For this review, take the finished solid that the model builds, in its own axes (mm). Face numbers are marked on the shaded views. Coordinates: 2 decimals unless noted, no trailing zeros. Loops run counter-clockwise (first coordinate to the right, second up) from the corner with the lowest first, then second, coordinate; pieces in that order, holes last. Notation, with made-up numbers: M 32,42 L 74,42 A34 cw 74,77 Z; hole C 42.25,16.25 d6. An arc over 180 degrees is marked long. Put each result on its own line as item: value.
Autodesk Inventor part; units mm, degrees
ref_plane "B1_XY" through (5.5, 0, 13.5) normal (1, 0, 0) x (0, 0, -1)
ref_plane "B1_YZ" through (5.5, 0, 13.5) normal (0, 0, -1) x (0, 1, 0)
ref_plane "B1_ZX" through (5.5, 0, 13.5) normal (0, 1, 0) x (1, 0, 0)
sketch "Sketch_1" plane through (0, 0, 0) normal (0, 0, 1) x (1, 0, 0)
  line L0 (5.5, 0) -> (-5.5, 0)
  line L1 (-5.5, 13.5) -> (-5.5, 9)
  line L2 (-5.5, 9) -> (-4.688, 8.188)
  line L3 (-4.688, 8.188) -> (4.688, 8.188)
  line L4 (4.688, 8.188) -> (5.5, 9)
  line L5 (5.5, 9) -> (5.5, 13.5)
  line L6 (5.5, 13.5) -> (3.7102, 16.6)
  line L7 (3.7102, 16.6) -> (-3.7102, 16.6)
  line L8 (-3.7102, 16.6) -> (-5.5, 13.5)
revolve "Revolution1" add sketch "Sketch_1" angle 360 about axis through (5.5, 0, 0) along (1, 0, 0)
thread "Thread1"
sketch "Sketch_2" plane through (0, 0, 0) normal (1, 0, 0) x (0, 1, 0)
  circle A0 centre (0, 0) radius 50
  line L0 (-7.7942, 13.5) -> (-15.5885, 0)
  line L1 (-15.5885, 0) -> (-7.7942, -13.5)
  line L2 (-7.7942, -13.5) -> (7.7942, -13.5)
  line L3 (7.7942, -13.5) -> (15.5885, 0)
  line L4 (15.5885, 0) -> (7.7942, 13.5)
  line L5 (7.7942, 13.5) -> (-7.7942, 13.5)
extrude "Extrusion1" cut sketch "Sketch_2" along normal mid plane 22
ref_plane "B1_XY" through (5.5, 0, 13.5) normal (1, 0, 0) x (0, 0, -1)
ref_plane "B1_YZ" through (5.5, 0, 13.5) normal (0, 0, -1) x (0, 1, 0)
ref_plane "B1_ZX" through (5.5, 0, 13.5) normal (0, 1, 0) x (1, 0, 0)
ref_plane "N_R_XY" through (0, 0, 0) normal (1, 0, 0) x (0, 0, -1)
ref_plane "N_R_YZ" through (0, 0, 0) normal (0, 0, -1) x (0, 1, 0)
ref_plane "N_R_ZX" through (0, 0, 0) normal (0, 1, 0) x (1, 0, 0)
properties part number "NT-05(63)_CE2"
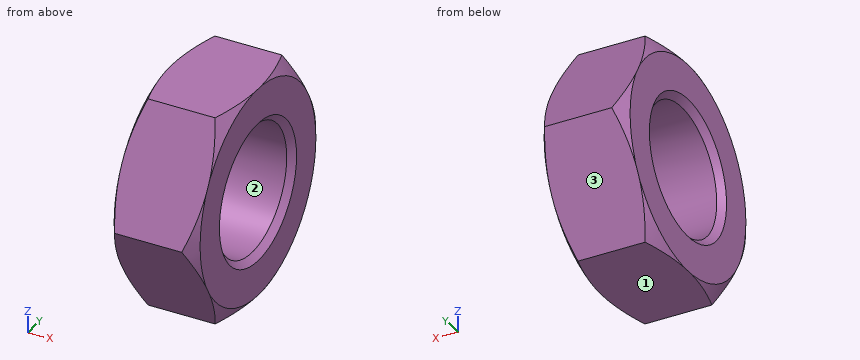
(1) Draft analysis for pull direction Y (two halves, no side actions). For the marked faces 1, 2 and 3, state which applies: +Y half, -Y half, draft (parallel to the pull), parting line (faces both ways), or undercut.
Determined:
face 1: draft
face 2: undercut
face 3: +Y half
(2) Add section A-A (x = 0). Write out the cut boundary in (y, z), plus the area to 3 significant figures.
Determined:
outline: M -15.59,0 L -7.79,-13.5 L 7.79,-13.5 L 15.59,0 L 7.79,13.5 L -7.79,13.5 Z; hole C 0,0 d16.38
area: 421 mm^2
(3) Wall thickness on line 1 along Z through (x, y) = (2, 0); line 2 along Y through (x, z) = (-1, -2.5); line 3 along Y through (x, z) = (-3, 7): over which ranges is each line inside the solid? List them lowest first. Write a range as [from, to].
Determined:
line 1: z = [-13.5, -8.19], [8.19, 13.5]
line 2: y = [-14.15, -7.8], [7.8, 14.15]
line 3: y = [-11.55, -4.25], [4.25, 11.55]
(4) For pin 1 (12 mm diameter, centred on y = -1, z = -8, fed in from -X); pin 2 (4 mm diameter, centred on x = -3.5, y = -11, fed in from -Z), all flat-tipped, find the tip position at first contact; note any pin that passes through.
Determined:
pin 1: stops at x = -5.5
pin 2: stops at z = -11.41
